Autodesk Inventor part; units mm, degrees
ref_plane "YZ Plane" through (0, 0, 0) normal (1, 0, 0) x (0, 1, 0)
ref_plane "XZ Plane" through (0, 0, 0) normal (0, 1, 0) x (-1, 0, 0)
ref_plane "XY Plane" through (0, 0, 0) normal (0, 0, 1) x (1, 0, 0)
sketch "Sketch2" plane through (0, 0, 0) normal (0, 1, 0) x (-1, 0, 0)
  line L0 (53, 48) -> (-53, 48)
  line L1 (-53, 48) -> (-53, -48)
  line L2 (-53, -48) -> (53, -48)
  line L3 (53, -48) -> (53, 48)
  line L4 (53, 48) -> (-53, -48) construction
  line L5 (-53, 48) -> (53, -48) construction
  point P0 (0, 0)
  dimension "d20" = 106
  dimension "d21" = 96
extrude "Extrusion1" add sketch "Sketch2" along normal blind 3
sketch "Sketch4" plane through (0, 3, 0) normal (0, 1, 0) x (1, 0, 0)
  line L0 (53, -48) -> (53, 48)
  line L1 (-53, -48) -> (53, -48)
  line L2 (53, 48) -> (50, 48)
  line L3 (50, 48) -> (50, -48)
  line L4 (50, -48) -> (53, -48)
  line L5 (53, -48) -> (53, 48)
  line L6 (53, 48) -> (-53, 48)
  line L7 (-53, 48) -> (-50, 48)
  line L8 (-50, 48) -> (-50, -48)
  line L9 (-50, -48) -> (-53, -48)
  line L10 (-53, -48) -> (-53, 48)
  point P0 (0, 0)
  dimension "d22" = 3
  dimension "d45" = 3
extrude "Extrusion3" add sketch "Sketch4" along normal blind 96 contours L1 L3 L2 L0 | L1 L10 L6 L8
sketch "Sketch5" plane through (53, 0, 48) normal (1, 0, 0) x (0, 0, -1)
  line L0 (48, 99) -> (48, 0) construction
  line L1 (0, 99) -> (96, 99)
  circle A0 centre (48, 49.5) radius 37.5
  dimension "d27" = 75
extrude "Extrusion4" cut sketch "Sketch5" against normal blind 164.2625
sketch "Sketch6" plane through (53, 0, 48) normal (1, 0, 0) x (0, 0, -1)
  circle A0 centre (48, 49.5) radius 37.5
  circle A1 centre (48, 49.5) radius 42 construction
  circle A2 centre (90, 49.5) radius 2
  circle A3 centre (48, 49.5) radius 42 construction
  circle A4 centre (77.6985, 79.1985) radius 2
  circle A5 centre (48, 49.5) radius 42 construction
  circle A6 centre (48, 91.5) radius 2
  circle A7 centre (48, 49.5) radius 42 construction
  circle A8 centre (18.3015, 79.1985) radius 2
  circle A9 centre (48, 49.5) radius 42 construction
  circle A10 centre (6, 49.5) radius 2
  circle A11 centre (48, 49.5) radius 42 construction
  circle A12 centre (18.3015, 19.8015) radius 2
  circle A13 centre (48, 49.5) radius 42 construction
  circle A14 centre (48, 7.5) radius 2
  circle A15 centre (48, 49.5) radius 42 construction
  circle A16 centre (77.6985, 19.8015) radius 2
  point P0 (48, 0)
  dimension "d30" = 84
  dimension "d31" = 4
  dimension "d34" = 360
extrude "Extrusion5" cut sketch "Sketch6" against normal blind 164.2625 contours A2 | A4 | A6 | A8 | A10 | A12 | A14 | A16
sketch "Sketch7" plane through (0, 0, 0) normal (0, -1, 0) x (1, 0, 0)
  line L0 (53, -48) -> (-53, -48)
  line L1 (0, -48) -> (0, -43) construction
  line L2 (0, -43) -> (0, -33) construction
  circle A0 centre (0, -43) radius 2
  circle A1 centre (0, -33) radius 2
  point P0 (0, 0)
  dimension "d38" = 5
  dimension "d39" = 10
  dimension "d40" = 4
  dimension "d41" = 4
extrude "Extrusion6" cut sketch "Sketch7" against normal blind 4
properties part number "shoulder"
Verification items for the finished model (mm, model axes). A direction names the side the tool comes from. Round coordinates to 2 decimals unless told otherwise and drop trailing zeros. Order: outer loops, then holes, each group sorted by start corner. A loop starts at its lowest first (then second) coordinate and runs counter-clockwise, first axis right, second up.
1. Access from +Z, -Z, +X, -X, +Y, -Y to the whole of each face (thin tool, end or side, straight path). Record for faces 1 (the cylindrical face through (-51.48, 19.04, -31.55)), 2 (the flat face through (1, 3, 1)).
Final values:
face 1: +X, -X
face 2: +Z, -Z, +Y
2. Section check B-B on z = 0. State how many separate pieces and enclosed holes the cut face has, then the cut area to 3 significant figures.
Final values:
separate pieces: 7
enclosed holes: 0
area: 396 mm2
3. Section check D-D on z = 16.5. Record the cut outline in (x, y), then the cut area to 3 significant figures.
Final values:
outline: (-53, 0) - (53, 0) - (53, 15.83) - (50, 15.83) - (50, 3) - (-50, 3) - (-50, 15.83) - (-53, 15.83) - close; (-53, 83.17) - (-50, 83.17) - (-50, 99) - (-53, 99) - close; (50, 83.17) - (53, 83.17) - (53, 99) - (50, 99) - close
area: 490 mm2
4. Thickness scan on L1, parallel to Y at x = -51.55, z = -42; L2, parallel to X at y = 27.5, z = 33; L3, parallel to Y at x = -19.5, z = -9. Record the ranges inside material, lowest first.
Final values:
L1: y = 0 to 47.5, 51.5 to 99
L2: x = -53 to -50, 50 to 53
L3: y = 0 to 3
5. Release check for a two-part mould opening along Z. For faces 3 (the flat face through (51, 99, -1)), 4 (the cylindrical face through (-51.48, 77.42, 28.78)), 5 (the flat face through (0, 2, -48)), 6 (the cylindrical face through (-51.479, 93.483, 0.26)) record: +Z half, -Z half, draft (parallel to the pull), parting line (faces both ways), or undercut.
Final values:
face 3: draft
face 4: undercut
face 5: -Z half
face 6: undercut
6. Go/stop test with flat-tipped pins: P1, Ø10, axis at x = -42, y = 71, coming from the -Z side; P2, Ø3, axis at x = 24, z = 19, coming from the +Y side; P3, Ø5, axis at y = 79.2, z = -29.7, coming from the +X side. Record where each tip stops, or that it passes through.
Final values:
P1: passes through
P2: stops at y = 3
P3: stops at x = 53
7. Section check A-A on y = 91.5. Record the cut outline in (x, z).
Final values:
outline: (-53, -48) - (-50, -48) - (-50, -2) - (-53, -2) - close; (-53, 2) - (-50, 2) - (-50, 48) - (-53, 48) - close; (50, -48) - (53, -48) - (53, -2) - (50, -2) - close; (50, 2) - (53, 2) - (53, 48) - (50, 48) - close
